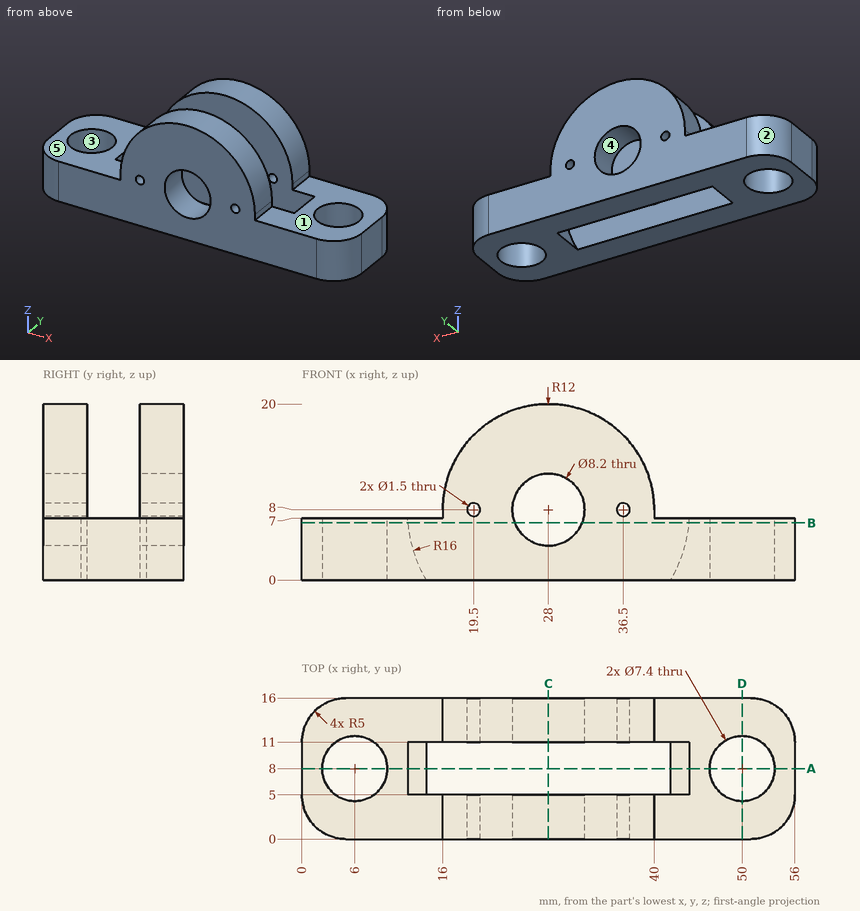
Design review of the part shown in the three views and the two pictorial views. Dimensions are in mm from the part's minimum x, y and z. A direction names the side the tool comes from. Round coordinates to 2 decimals unless told otherwise and drop trailing zeros. Write each loop counter-clockwise with the first axis right and the second up, starting at its lowest first coordinate (ties: lowest second). Pieces come first, ordered by that corner, then holes. Notation, with made-up numbers: (48.25, 14.5) - (107.25, 14.5) arc R10 ccw to (107.25, 21.5) - close; hole circle Ø9 at (-38, 10). An arc over 180 degrees is marked (long way). Answer as CSV lines item,"result". Start each with the question number.
(1) Add section B-B, the plane z = 6.5. State the section outline as (x, y) points, plus the area to 3 significant figures.
(2) Add section C-C, the plane x = 28. State the section outline as (y, z) points.
(3) Add section A-A, the plane y = 8. State the section outline as (x, z) points, plus the area to 3 significant figures.
(4) Machinability: for the marked faces 1 and 2, which of the approach directions +Z, -Z, +X, -X, +Y, -Y give a long, thin tool a straight path to every point of the face, cutting with its end or side? Answer none if there is none.
(5) For line 1 (Y direction, x = 34.5, z = 15.5); line 2 (Y direction, x = 50, z = 5); line 3 (X direction, y = 10.75, z = 1), list the stretches that pass through material, from the lowest coordinate up.
(6) For pin 1 (6 mm diameter, centred on x = 6, y = 8, fed in from +Z); pin 2 (5 mm diameter, centred on x = 50.5, y = 4.5, fed in from +Z); pin 3 (8 mm diameter, centred on x = 13.5, y = 3, fed in from +Z); pin 4 (0.5 mm diameter, centred on y = 3.5, z = 7.5, fed in from +X), all flat-tipped, find the tip position at first contact; note any pin that passes through.
(7) Mouldability with a two-part tool opening along Z and no side actions: class the marked faces 3, 4 and 5 as +Z half, -Z half, draft (parallel to the pull), parting line (faces both ways), or undercut.
(8) Add section D-D, the plane x = 50. State the section outline as (y, z) points, plus the area to 3 significant figures.
From the geometry:
1,outline,"(0, 5) arc R5 ccw to (5, 0) - (24.18, 0) - (24.18, 5) - (12.07, 5) - (12.07, 11) - (24.18, 11) - (24.18, 16) - (5, 16) arc R5 ccw to (0, 11) - close; (31.82, 0) - (51, 0) arc R5 ccw to (56, 5) - (56, 11) arc R5 ccw to (51, 16) - (31.82, 16) - (31.82, 11) - (43.93, 11) - (43.93, 5) - (31.82, 5) - close; hole circle Ø7.4 at (6, 8); hole circle Ø7.4 at (50, 8)"
1,area,"521 mm²"
2,outline,"(0, 0) - (5, 0) - (5, 3.9) - (0, 3.9) - close; (0, 12.1) - (5, 12.1) - (5, 20) - (0, 20) - close; (11, 0) - (16, 0) - (16, 3.9) - (11, 3.9) - close; (11, 12.1) - (16, 12.1) - (16, 20) - (11, 20) - close"
3,outline,"(0, 0) - (2.3, 0) - (2.3, 7) - (0, 7) - close; (9.7, 0) - (14.14, 0) arc R16 cw to (12.03, 7) - (9.7, 7) - close; (41.86, 0) - (46.3, 0) - (46.3, 7) - (43.97, 7) arc R16 cw to start; (53.7, 0) - (56, 0) - (56, 7) - (53.7, 7) - close"
3,area,"75.5 mm²"
4,face 1,"+Z, +X, +Y, -Y"
4,face 2,"+Z, -Z, -X, +Y"
5,line 1,"y = 0 to 5, 11 to 16"
5,line 2,"y = 0 to 4.3, 11.7 to 16"
5,line 3,"x = 0 to 3.52, 8.48 to 13.61, 42.39 to 47.52, 52.48 to 56"
6,pin 1,"passes through"
6,pin 2,"stops at z = 7"
6,pin 3,"stops at z = 13.81"
6,pin 4,"stops at x = 40"
7,face 3,"draft"
7,face 4,"undercut"
7,face 5,"+Z half"
8,outline,"(0, 0) - (4.3, 0) - (4.3, 7) - (0, 7) - close; (11.7, 0) - (16, 0) - (16, 7) - (11.7, 7) - close"
8,area,"60.2 mm²"
